Design review of the part built by this model. Coordinates are the model's own, in mm. Face numbers are marked on the shaded views. A direction names the side the tool comes from. Give positions to 0.01 mm unless a question says otherwise; leave off trailing zeros. Loops run counter-clockwise (first coordinate to the right, second up) from the corner with the lowest first, then second, coordinate; pieces in that order, holes last. Notation, with made-up numbers: (60, 89) -> (110, 89) arc R35 ccw to (110, 123) -> close; hole circle Ø10 at (62.25, 63.25). An arc over 180 degrees is marked (long way). Use a Markdown table: item, result. Add a question column.
1. For pin 1 Ø12 at (x, y) = (-13, 2.5) entering from +Z; pin 2 Ø8 at (x, y) = (4, 35.75) entering from +Z; pin 3 Ø1.5 at (x, z) = (-19, 3) entering from +Y, all flat-tipped, find the tip position at first contact; note any pin that passes through.
2. Add section C-C (z = 2.25). State the section outline as (x, y) points, and give its area (3 significant figures).
3. To check wall thickness, follow line 1 (Y direction, x = 4, z = 3); line 2 (Y direction, x = 6, z = 2); line 3 (Z direction, x = -21, y = 1.7). State the ranges of each line that lie inside material, in increasing order.
4. Add section D-D (y = -18). State the section outline as (x, z) points.
5. Add section A-A (y = -2). State the section outline as (x, z) points.
6. For the marked faces 1, 2 and 3, list the 3-axis set-ups (+Z, -Z, +X, -X, +Y, -Y) from which the entire face can be reached by the end or side of a thin tool; tool diameter is ignored.
7. Draft analysis for pull direction Y (two halves, no side actions). For the marked faces 4, 5 and 6, state which applies: pulls with the +Y half, pulls with the -Y half, needs draft (parallel to the pull), parting line crosses it, or undercut.
8. Add section B-B (z = 5.75). State the section outline as (x, y) points, and give its area (3 significant figures).
```python
from build123d import *

# Parameters (mm, degrees)
F0_R          = 2.5
F1_DEPTH      = 5
F2_R          = 5
F3_DEPTH      = 4
F3_DEPTH_BACK = 4
F4_R          = 1.75
F5_DEPTH      = 39.751
F5_DEPTH_BACK = 39.751
F6_SIZE       = 0.5


# Not quite as in the source:
# - after a boolean that leaves OpenCascade's solid faulty, fix() repairs it


with BuildPart() as f1:
    # F0 (on Top) → F1 (new body)
    with BuildSketch(Plane.XY):
        with BuildLine():
            Line((-16, 4), (-26, 4))
            Line((-26, 4), (-26, 0))
            Line((-26, 0), (-26, -4))
            Line((-26, -4), (-16, -4))
            ThreePointArc((-16, -4), (-8.9289321881, -6.9289321881), (-6, -14))
            Line((-6, -14), (-6, -35.75))
            ThreePointArc((-6, -35.75), (-4.8284271247, -38.5784271247), (-2, -39.75))
            Line((-2, -39.75), (4, -39.75))
            ThreePointArc((4, -39.75), (8, -35.75), (4, -31.75))
            ThreePointArc((4, -31.75), (1.1715728753, -30.5784271247), (0, -27.75))
            Line((0, -27.75), (0, 0))
            Line((0, 0), (0, 27.75))
            ThreePointArc((0, 27.75), (1.1715728753, 30.5784271247), (4, 31.75))
            ThreePointArc((4, 31.75), (8, 35.75), (4, 39.75))
            Line((4, 39.75), (-2, 39.75))
            ThreePointArc((-2, 39.75), (-4.8284271247, 38.5784271247), (-6, 35.75))
            Line((-6, 35.75), (-6, 14))
            ThreePointArc((-6, 14), (-8.9289321881, 6.9289321881), (-16, 4))
        make_face()
        with Locations((4, -35.75)):
            Circle(F0_R, mode=Mode.SUBTRACT)
        with Locations((4, 35.75)):
            Circle(F0_R, mode=Mode.SUBTRACT)
    extrude(amount=F1_DEPTH)

    # F2 (on Front) → F3 (join, two sides)
    with BuildSketch(Plane.XZ) as f3_sk:
        with Locations((-21, 5)):
            Circle(F2_R)
    extrude(amount=F3_DEPTH)
    extrude(f3_sk.sketch, amount=-F3_DEPTH_BACK)

    # F4 (on Front) → F5 (cut, two sides)
    with BuildSketch(Plane.XZ) as f5_sk:
        with BuildLine():
            ThreePointArc((-21, 0), (-24.5355339059, 1.4644660941), (-26, 5))
            Line((-26, 5), (-26, 0))
            Line((-26, 0), (-21, 0))
        make_face()
        with Locations((-21, 5)):
            Circle(F4_R)
    extrude(amount=-F5_DEPTH, mode=Mode.SUBTRACT)
    extrude(f5_sk.sketch, amount=F5_DEPTH_BACK, mode=Mode.SUBTRACT)

    add(f1.part.fix(), mode=Mode.REPLACE)

    # F6
    f6_edges = [f1.edges().sort_by_distance(p)[0] for p in [
        (1.5, 35.75, 5),
        (1.5, -35.75, 5),
    ]]
    chamfer(f6_edges, length=F6_SIZE)


solid = f1.part
```
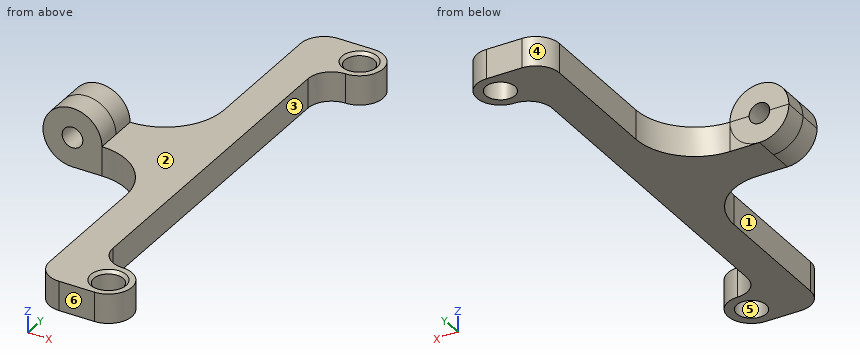
Taken from the geometry:
| question | item | result |
|---|---|---|
| 1 | pin 1 | stops at z = 9.58 |
| 1 | pin 2 | stops at z = 5 |
| 1 | pin 3 | stops at y = 4 |
| 2 | outline | (-25.18, -4) -> (-16, -4) arc R10 cw to (-6, -14) -> (-6, -35.75) arc R4 ccw to (-2, -39.75) -> (4, -39.75) arc R4 ccw to (4, -31.75) arc R4 cw to (0, -27.75) -> (0, 27.75) arc R4 cw to (4, 31.75) arc R4 ccw to (4, 39.75) -> (-2, 39.75) arc R4 ccw to (-6, 35.75) -> (-6, 14) arc R10 cw to (-16, 4) -> (-25.18, 4) -> close; hole circle Ø5 at (4, -35.75); hole circle Ø5 at (4, 35.75) |
| 2 | area | 748 mm^2 |
| 3 | line 1 | y = -39.75 to -38.25, -33.25 to -31.75, 31.75 to 33.25, 38.25 to 39.75 |
| 3 | line 2 | y = -39.21 to -37.25, -34.25 to -32.29, 32.29 to 34.25, 37.25 to 39.21 |
| 3 | line 3 | z = 0 to 3.25, 6.75 to 10 |
| 4 | outline | (-6, 0) -> (0, 0) -> (0, 5) -> (-6, 5) -> close |
| 5 | outline | (-21, 0) -> (0, 0) -> (0, 5) -> (-16, 5) arc R5 ccw (long way) to start; hole circle Ø3.5 at (-21, 5) |
| 6 | face 1 | +Z, -Z, -X, -Y |
| 6 | face 2 | +Z, +X, +Y, -Y |
| 6 | face 3 | +Z, -Z, +X |
| 7 | face 4 | pulls with the +Y half |
| 7 | face 5 | undercut |
| 7 | face 6 | pulls with the -Y half |
| 8 | outline | (-25.94, -4) -> (-22.58, -4) -> (-22.58, 4) -> (-25.94, 4) -> close; (-19.42, -4) -> (-16.06, -4) -> (-16.06, 4) -> (-19.42, 4) -> close |
| 8 | area | 53.8 mm^2 |
